```python
from build123d import *

# Parameters (mm, degrees)
SKETCH016_W     = 30
SKETCH016_H     = 70
PAD006_DEPTH    = 5
FILLET007_R     = 10
SKETCH017_W     = 30
SKETCH017_H     = 30.4
POCKET018_DEPTH = 2
FILLET008_R     = 2
FILLET009_R     = 2
SKETCH018_R     = 1.25
POCKET019_DEPTH = 9
SKETCH019_R     = 2
POCKET020_DEPTH = 1.5


with BuildPart() as part:
    # Sketch016 → Pad006 (new body)
    with BuildSketch(Plane.XZ):
        Rectangle(SKETCH016_W, SKETCH016_H)
    extrude(amount=PAD006_DEPTH)

    # Fillet007
    fillet007_edges = [part.edges().sort_by_distance(p)[0] for p in [
        (15, -2.5, -35),
        (-15, -2.5, -35),
        (15, -2.5, 35),
        (-15, -2.5, 35),
    ]]
    fillet(fillet007_edges, radius=FILLET007_R)

    # Sketch017 (on Face2 of Fillet007) → Pocket018 (cut)
    with BuildSketch(Plane(origin=(0, 0, 0), x_dir=(1, 0, 0), z_dir=(0, 1, 0))):
        Rectangle(SKETCH017_W, SKETCH017_H)
    extrude(amount=-POCKET018_DEPTH, mode=Mode.SUBTRACT)

    # Fillet008
    fillet008_edges = [part.edges().sort_by_distance(p)[0] for p in [
        (15, -2, 0),
        (-15, -2, 0),
    ]]
    fillet(fillet008_edges, radius=FILLET008_R)

    # Fillet009
    fillet009_edges = [part.edges().sort_by_distance(p)[0] for p in [
        (15, 0, -20.1),
        (15, 0, 20.1),
    ]]
    fillet(fillet009_edges, radius=FILLET009_R)

    # Sketch018 (on Face4 of Fillet009) → Pocket019 (cut)
    with BuildSketch(Plane.XZ.offset(5)):
        Circle(SKETCH018_R)
    extrude(amount=-POCKET019_DEPTH, mode=Mode.SUBTRACT)

    # Sketch019 (on Face4 of Pocket019) → Pocket020 (cut)
    with BuildSketch(Plane.XZ.offset(5)):
        Circle(SKETCH019_R)
    extrude(amount=-POCKET020_DEPTH, mode=Mode.SUBTRACT)


with BuildPart() as part_1:
    # Body003 placement: moved
    add(part.part.moved(Location((-0.25, -90.79, -8.4))))


solid = part_1.part
```
The model under review builds one solid part; all positions refer to its coordinate system, in mm. A direction names the side the tool comes from. Round coordinates to 2 decimals unless told otherwise and drop trailing zeros. Loops run counter-clockwise (first coordinate to the right, second up) from the corner with the lowest first, then second, coordinate; pieces in that order, holes last. Notation, with made-up numbers: (78, -14.75) - (136, -14.75) arc R16 cw to (136, 1.25) - close; hole circle Ø1 at (51, 74.25). An arc over 180 degrees is marked (long way). Write each question's results on one line, items separated by ' | '. Start each with the question number.
Q1. Insertion check: P1, Ø3, axis at x = -0.25, z = -8.4, coming from the +Y side; P2, Ø3.5, axis at x = -0.25, z = -8.4, coming from the -Y side; P3, Ø1.5, axis at y = -93, z = -4.5, coming from the -X side. Each pin has a flat end and moves straight along its axis. Give the tip position at first contact, or say it passes through.
Q2. Take a section at B-B on z = -8.4. Give the boundary of the cut face in (x, y), plus the area to 3 significant figures.
Q3. Tool access review of faces 5 (the cylindrical face through (14.15, -93.36, -8.61)), 6 (the cylindrical face through (-12.4, -94.31, -40.39)), 7 (the flat face through (0, -94.29, -10)): name each direction out of +Z, -Z, +X, -X, +Y, -Y from which nothing blocks a thin tool from reaching the whole face with its end or side.
Q4. Wall thickness on line 1 along Z through (x, y) = (-0.25, -94.65); line 2 along Z through (x, y) = (-1, -92.6); line 3 along Y through (x, z) = (9, 23.5): over which ranges is each line inside the solid? List them lowest first. Write a range as [from, to].
Q5. Take a section at A-A on x = -0.25. Give the boundary of the cut face in (y, z), plus the area to 3 significant figures.
Q6. Draft analysis for pull direction X (two halves, no side actions). For faces 1 (the flat face through (-3, -92.79, -9)), 2 (the cylindrical face through (-14.68, -91.39, -28.57)), 3 (the cylindrical face through (14.15, -91.36, 11.77)), 4 (the cylindrical face through (-0.51, -95.05, -6.417)), state which applies: pulls with the +X half, pulls with the -X half, needs draft (parallel to the pull), parting line crosses it, or undercut.
Q7. Take a section at C-C on z = -21. Give the boundary of the cut face in (x, y).
Data:
1) P1: stops at y = -92.79 | P2: stops at y = -94.29 | P3: stops at x = -14.96
2) outline: (-15.25, -95.79) - (-2.25, -95.79) - (-2.25, -94.29) - (-1.5, -94.29) - (-1.5, -92.79) - (-13.25, -92.79) arc R2 ccw to (-15.25, -94.79) - close; (1, -94.29) - (1.75, -94.29) - (1.75, -95.79) - (14.75, -95.79) - (14.75, -94.79) arc R2 ccw to (12.75, -92.79) - (1, -92.79) - close | area: 78.5 mm²
3) face 5: +X, +Y | face 6: -Z, -X, +Y, -Y | face 7: -Y
4) line 1: z = [-43.4, -10.4], [-6.4, 26.6] | line 2: z = [-43.39, -23.6], [6.8, 26.59] | line 3: y = [-95.79, -90.79]
5) outline: (-95.79, -43.4) - (-92.79, -43.4) arc R2 ccw to (-90.79, -41.4) - (-90.79, -23.6) - (-92.79, -23.6) - (-92.79, -9.65) - (-94.29, -9.65) - (-94.29, -10.4) - (-95.79, -10.4) - close; (-95.79, -6.4) - (-94.29, -6.4) - (-94.29, -7.15) - (-92.79, -7.15) - (-92.79, 6.8) - (-90.79, 6.8) - (-90.79, 24.6) arc R2 ccw to (-92.79, 26.6) - (-95.79, 26.6) - close | area: 278 mm²
6) face 1: needs draft | face 2: pulls with the -X half | face 3: pulls with the +X half | face 4: undercut
7) outline: (-15.25, -95.79) - (14.75, -95.79) - (14.75, -94.79) arc R2 ccw to (12.75, -92.79) - (-13.25, -92.79) arc R2 ccw to (-15.25, -94.79) - close
